For this review, take the finished solid that the model builds, in its own axes (mm). A direction names the side the tool comes from. Coordinates: 2 decimals unless noted, no trailing zeros. Write each loop counter-clockwise with the first axis right and the second up, starting at its lowest first coordinate (ties: lowest second). Pieces come first, ordered by that corner, then holes. Notation, with made-up numbers: (-39, 11.5) -> (10, 11.5) arc R21 ccw to (10, 49.5) -> close; hole circle Ø3 at (-38.75, -13). An arc over 180 degrees is marked (long way). One line per item, written item: value. Start each with the question number.
1) Mouldability with a two-part tool opening along X and no side actions: class faces 3 (the flat face through (0, 3, 11)), 4 (the cylindrical face through (10.91, 4.01, 30.47)), 5 (the flat face through (20, 5, 8)) as released by +X, released by -X, zero draft, split by the parting line, or undercut.
2) Machinability: for faces 1 (the cylindrical face through (30.91, 4.01, 30.47)), 2 (the cylindrical face through (31.85, 1.521, 28.284)), which of the approach directions +Z, -Z, +X, -X, +Y, -Y give a long, thin tool a straight path to every point of the face, cutting with its end or side? Answer none if there is none.
3) For probe 1 along Z at (x, y) = (10.45, 4.05); probe 2 along Z at (x, y) = (10.45, 0.85); probe 3 along X at (y, z) = (1.95, 28), list the stretches that pass through material, from the lowest coordinate up. Write a range as from..to.
4) For pin 1 Ø2 at (x, z) = (30, 5) entering from +Y; pin 2 Ø3.5 at (x, z) = (10.5, 3) entering from +Y, all flat-tipped, find the tip position at first contact; note any pin that passes through.
5) Add section A-A (x = 30.45). State the section outline as (y, z) points, and give its area (3 significant figures).
6) Add section B-B (y = 0.85). State the section outline as (x, z) points, and give its area (3 significant figures).
from build123d import *

# Parameters (mm, degrees)
BOSS_EXTRU_1_DEPTH      = 9
BOSS_EXTRU_1_DEPTH_BACK = 9
ESQUISSE1_W             = 8
ESQUISSE1_H             = 25
ESQUISSE1_R             = 2
ESQUISSE1_W_2           = 40.9
ESQUISSE1_H_2           = 5
ESQUISSE2_W             = 40.9
ESQUISSE2_H             = 7
ESQUISSE2_H_2           = 23
BOSS_EXTRU_2_DEPTH      = 5
ESQUISSE5_W             = 8
ESQUISSE5_H             = 18
ENL_V_MAT_EXTRU_2_DEPTH = 64.562646263
ESQUISSE6_R             = 1.9
ENL_V_MAT_EXTRU_3_DEPTH = 10
CONG_1_R                = 5
ESQUISSE7_R             = 3.5
ENL_V_MAT_EXTRU_4_DEPTH = 2


with BuildPart() as part:
    # Esquisse1 → Boss.-Extru.1 (new, two sides: drawn at the far end of the back side and taken through both)
    # profile 1 of 3: a face of its own
    with BuildSketch(Plane.XY.offset(-BOSS_EXTRU_1_DEPTH_BACK)):
        with Locations((-4, 12.5)):
            Rectangle(ESQUISSE1_W, ESQUISSE1_H)
        with Locations((-3.85, 10)):
            Circle(ESQUISSE1_R, mode=Mode.SUBTRACT)
        with Locations((-3.85, 20)):
            Circle(ESQUISSE1_R, mode=Mode.SUBTRACT)
    # profile 2 of 3: a face of its own
    with BuildSketch(Plane.XY.offset(-BOSS_EXTRU_1_DEPTH_BACK)):
        with Locations((20.45, 2.5)):
            Rectangle(ESQUISSE1_W_2, ESQUISSE1_H_2)
    # profile 3 of 3: a face of its own
    with BuildSketch(Plane.XY.offset(-BOSS_EXTRU_1_DEPTH_BACK)):
        with Locations((44.9, 12.5)):
            Rectangle(ESQUISSE1_W, ESQUISSE1_H)
        with Locations((44.75, 10)):
            Circle(ESQUISSE1_R, mode=Mode.SUBTRACT)
        with Locations((44.75, 20)):
            Circle(ESQUISSE1_R, mode=Mode.SUBTRACT)
    extrude(amount=BOSS_EXTRU_1_DEPTH + BOSS_EXTRU_1_DEPTH_BACK)

    # Esquisse2 → Boss.-Extru.2 (add)
    with BuildSketch(Plane(origin=(0, 5, 0), x_dir=(1, 0, 0), z_dir=(0, 1, 0))):
        with Locations((20.45, 12.5)):
            Rectangle(ESQUISSE2_W, ESQUISSE2_H)
        with Locations((20.45, -20.5)):
            Rectangle(ESQUISSE2_W, ESQUISSE2_H_2)
    extrude(amount=-BOSS_EXTRU_2_DEPTH)

    # Esquisse5 → Enl_v. mat.-Extru.2 (cut, through all)
    with BuildSketch(Plane(origin=(0, 25, 0), x_dir=(1, 0, 0), z_dir=(0, 1, 0))):
        with Locations((-4, 0)):
            Rectangle(ESQUISSE5_W, ESQUISSE5_H)
        with Locations((44.9, 0)):
            Rectangle(ESQUISSE5_W, ESQUISSE5_H)
    extrude(amount=-ENL_V_MAT_EXTRU_2_DEPTH, mode=Mode.SUBTRACT)

    # Esquisse6 → Enl_v. mat.-Extru.3 (cut)
    with BuildSketch(Plane(origin=(0, 5, 0), x_dir=(1, 0, 0), z_dir=(0, 1, 0))):
        with Locations(Location((10.45, -4.5, 0), (0, 0, 180))):
            Circle(ESQUISSE6_R)
        with Locations(Location((30.45, -4.5, 0), (0, 0, 180))):
            Circle(ESQUISSE6_R)
        with Locations(Location((10.45, -27, 0), (0, 0, 180))):
            Circle(ESQUISSE6_R)
        with Locations(Location((30.45, -27, 0), (0, 0, 180))):
            Circle(ESQUISSE6_R)
    extrude(amount=-ENL_V_MAT_EXTRU_3_DEPTH, mode=Mode.SUBTRACT)

    # Cong_1
    cong_1_edges = [part.edges().sort_by_distance(p)[0] for p in [
        (0, 2.5, -16),
        (40.9, 2.5, -16),
    ]]
    fillet(cong_1_edges, radius=CONG_1_R)

    # Esquisse7 → Enl_v. mat.-Extru.4 (cut)
    with BuildSketch(Plane(origin=(0, 5, 0), x_dir=(1, 0, 0), z_dir=(0, 1, 0))):
        with Locations(Location((10.45, -4.5, 0), (0, 0, 180))):
            Circle(ESQUISSE7_R)
        with Locations(Location((30.45, -4.5, 0), (0, 0, 180))):
            Circle(ESQUISSE7_R)
        with Locations(Location((30.45, -27, 0), (0, 0, 180))):
            Circle(ESQUISSE7_R)
        with Locations(Location((10.45, -27, 0), (0, 0, 180))):
            Circle(ESQUISSE7_R)
    extrude(amount=-ENL_V_MAT_EXTRU_4_DEPTH, mode=Mode.SUBTRACT)


solid = part.part
Numbers:
1. face 3: released by -X
1. face 4: undercut
1. face 5: zero draft
2. face 1: +Y
2. face 2: +Y, -Y
3. probe 1: -16..1, 8..23.5, 30.5..32
3. probe 2: -16..2.6, 6.4..25.1, 28.9..32
3. probe 3: 0..8.83, 12.07..28.83, 32.07..40.9
4. pin 1: through
4. pin 2: y = 3
5. outline: (0, -16) -> (5, -16) -> (5, 1) -> (3, 1) -> (3, 2.6) -> (0, 2.6) -> close; (0, 6.4) -> (3, 6.4) -> (3, 8) -> (5, 8) -> (5, 23.5) -> (3, 23.5) -> (3, 25.1) -> (0, 25.1) -> close; (0, 28.9) -> (3, 28.9) -> (3, 30.5) -> (5, 30.5) -> (5, 32) -> (0, 32) -> close
5. area: 189 mm²
6. outline: (0, -11) arc R5 ccw to (5, -16) -> (35.9, -16) arc R5 ccw to (40.9, -11) -> (40.9, 32) -> (0, 32) -> close; hole circle Ø3.8 at (10.45, 4.5); hole circle Ø3.8 at (10.45, 27); hole circle Ø3.8 at (30.45, 4.5); hole circle Ø3.8 at (30.45, 27)
6. area: 1,910 mm²
